Input: part model. Units: mm. Frame: model coordinates. Coordinates: 2 decimals unless noted, no trailing zeros. Loops run counter-clockwise (first coordinate to the right, second up) from the corner with the lowest first, then second, coordinate; pieces in that order, holes last. Notation, with made-up numbers: (50.25, 31.25) -> (90.25, 31.25) arc R12 cw to (90.25, 39.25) -> close; hole circle Ø10 at (32, -39). An arc over 180 degrees is marked (long way). Answer as a JSON object with one key per item and string values.
from build123d import *

# Parameters (mm, degrees)
SKETCH1_R           = 5.5
BOSS_EXTRUDE1_DEPTH = 2


with BuildPart() as part:
    # Sketch1 → Boss-Extrude1 (new body)
    with BuildSketch(Plane.XY):
        with BuildLine():
            Line((103.180041152, 46.419753086), (-196.819958848, 46.419753086))
            Line((-196.819958848, 46.419753086), (-196.819958848, -23.580246914))
            Line((-196.819958848, -23.580246914), (-157.819958848, -23.580246914))
            Line((-157.819958848, -23.580246914), (-157.819958848, 11.419753086))
            ThreePointArc((-157.819958848, 11.419753086), (-151.819958848, 17.419753086), (-145.819958848, 11.419753086))
            Line((-145.819958848, 11.419753086), (-145.819958848, -23.580246914))
            Line((-145.819958848, -23.580246914), (52.180041152, -23.580246914))
            Line((52.180041152, -23.580246914), (52.180041152, 11.419753086))
            ThreePointArc((52.180041152, 11.419753086), (58.180041152, 17.419753086), (64.180041152, 11.419753086))
            Line((64.180041152, 11.419753086), (64.180041152, -23.580246914))
            Line((64.180041152, -23.580246914), (103.180041152, -23.580246914))
            Line((103.180041152, -23.580246914), (103.180041152, 46.419753086))
        make_face()
        with Locations((-96.819958848, 21.296296296)):
            Circle(SKETCH1_R, mode=Mode.SUBTRACT)
        with Locations((3.180041152, 21.296296296)):
            Circle(SKETCH1_R, mode=Mode.SUBTRACT)
    extrude(amount=BOSS_EXTRUDE1_DEPTH)


solid = part.part
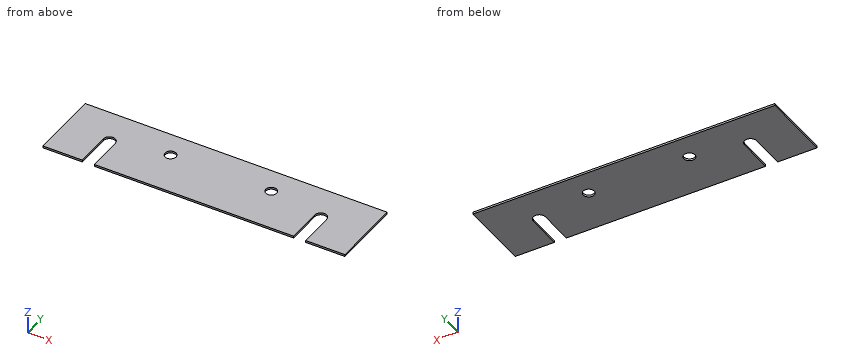
1. Section query B-B (x = 57). Return loops of the section in (y, z).
Reply:
{"outline": "(17.3, 0) -> (46.42, 0) -> (46.42, 2) -> (17.3, 2) -> close"}
2. Line query: line 1 along X through (y, z) = (-10.5, 0.2); line 2 along X through (y, z) = (22, 1.5); line 3 along X through (y, z) = (16.5, 1.35). Output: solid intervals per line, ascending.
Reply:
{"line 1": "x = -196.82 to -157.82, -145.82 to 52.18, 64.18 to 103.18", "line 2": "x = -196.82 to -102.27, -91.37 to -2.27, 8.63 to 103.18", "line 3": "x = -196.82 to -155.01, -148.63 to -99.51, -94.13 to 0.49, 5.87 to 54.99, 61.37 to 103.18"}
3. Section query A-A (z = 0.75). Return loops of the section in (x, y), plus the area to 3 significant figures.
Reply:
{"outline": "(-196.82, -23.58) -> (-157.82, -23.58) -> (-157.82, 11.42) arc R6 cw to (-145.82, 11.42) -> (-145.82, -23.58) -> (52.18, -23.58) -> (52.18, 11.42) arc R6 cw to (64.18, 11.42) -> (64.18, -23.58) -> (103.18, -23.58) -> (103.18, 46.42) -> (-196.82, 46.42) -> close; hole circle Ø11 at (-96.82, 21.3); hole circle Ø11 at (3.18, 21.3)", "area": "19,900 mm2"}
4. Pin query (flat end, axial travel): P1, Ø10, axis at x = 3.18, y = 21.3, coming from the -Z side. Return the tip coordinate at first contact, or that it passes through.
Reply:
{"P1": "passes through"}
